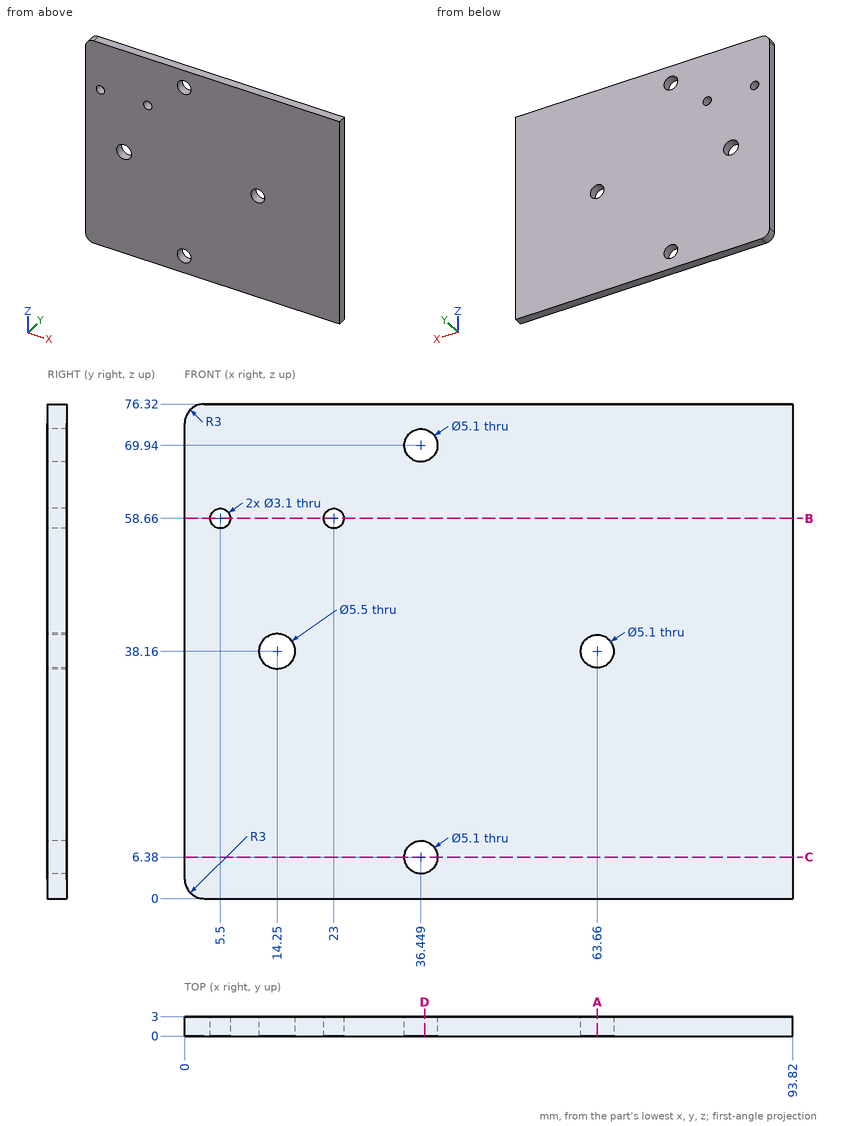
Drawing for the job (mm, zero at the part's lowest x, y, z). Round coordinates to 2 decimals unless told otherwise and drop trailing zeros. Loops run counter-clockwise (first coordinate to the right, second up) from the corner with the lowest first, then second, coordinate; pieces in that order, holes last. Notation, with made-up numbers: (-10, -19.5) - (37, -19.5) arc R24 cw to (37, 9.5) - close; hole circle Ø8 at (80.25, 20.25). An arc over 180 degrees is marked (long way). Write each question's results on one line, items separated by ' | '.
(1) Wall check: L1, parallel to Z at x = 63.66, y = 0.9; L2, parallel to Z at x = 5.5, y = 1.55; L3, parallel to Z at x = 34.5, y = 1.5. Give the ranges that are in metal, low to high.
Answer below:
L1: z = 0 to 35.61, 40.71 to 76.32 | L2: z = 0 to 57.11, 60.21 to 76.32 | L3: z = 0 to 4.74, 8.02 to 68.3, 71.58 to 76.32
(2) Saw through at B-B, the plane z = 58.66. List the corners of the cut face in (x, y).
Answer below:
outline: (0, 0) - (3.95, 0) - (3.95, 3) - (0, 3) - close; (7.05, 0) - (21.45, 0) - (21.45, 3) - (7.05, 3) - close; (24.55, 0) - (93.82, 0) - (93.82, 3) - (24.55, 3) - close
(3) Saw through at D-D, the plane x = 37. List the corners of the cut face in (y, z).
Answer below:
outline: (0, 0) - (3, 0) - (3, 3.89) - (0, 3.89) - close; (0, 8.87) - (3, 8.87) - (3, 67.45) - (0, 67.45) - close; (0, 72.43) - (3, 72.43) - (3, 76.32) - (0, 76.32) - close
(4) Saw through at C-C, the plane z = 6.38. List the corners of the cut face in (x, y), then the cut area to 3 significant figures.
Answer below:
outline: (0, 0) - (33.9, 0) - (33.9, 3) - (0, 3) - close; (39, 0) - (93.82, 0) - (93.82, 3) - (39, 3) - close | area: 266 mm^2
(5) Pin check, flat tips, straight feed: pin 1 (2 mm diameter, centred on x = 28.5, z = 21, fed in from -Y); pin 2 (3.5 mm diameter, centred on x = 14.25, z = 38.16, fed in from -Y). Stop position of each tip, or through.
Answer below:
pin 1: stops at y = 0 | pin 2: passes through
(6) Saw through at A-A, the plane x = 63.66. List the corners of the cut face in (y, z), then the cut area to 3 significant figures.
Answer below:
outline: (0, 0) - (3, 0) - (3, 35.61) - (0, 35.61) - close; (0, 40.71) - (3, 40.71) - (3, 76.32) - (0, 76.32) - close | area: 214 mm^2
